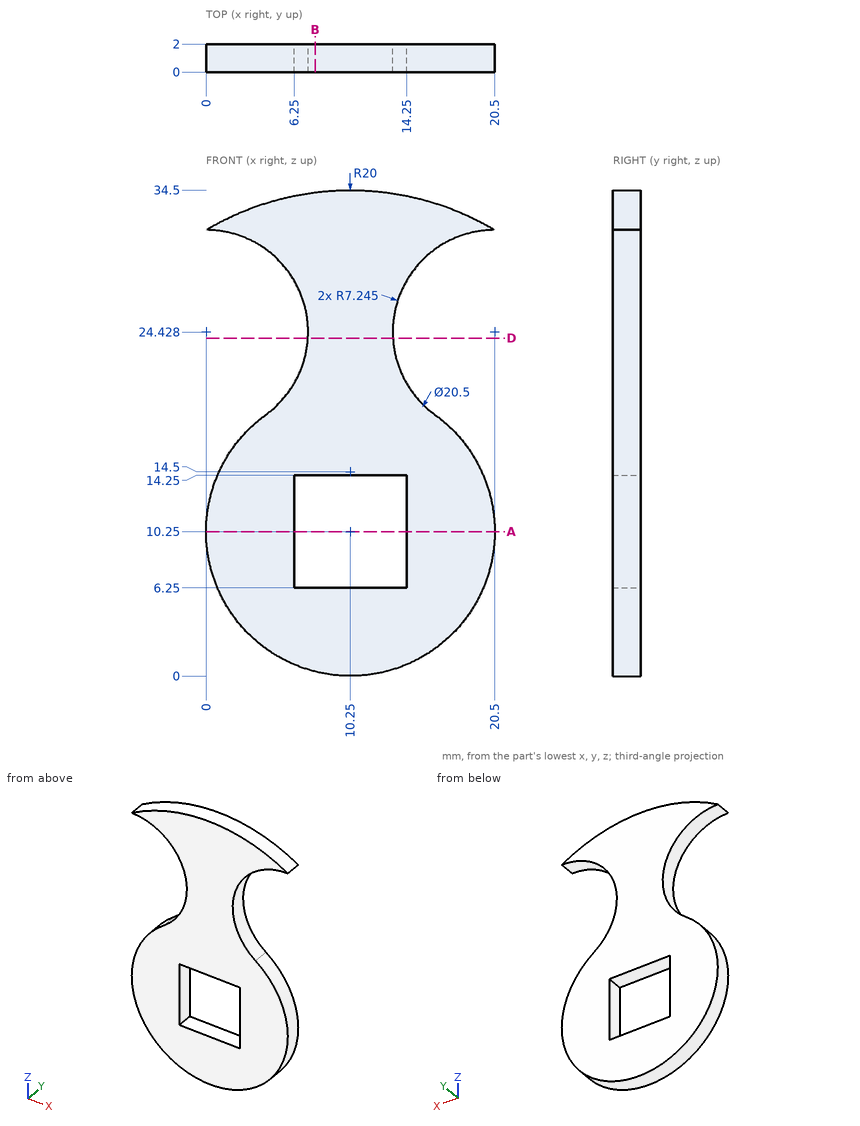
Source: three-view drawing plus pictorial views. Frame: mm from the lowest corner of the part. Round coordinates to 2 decimals unless told otherwise and drop trailing zeros. Order: outer loops, then holes, each group sorted by start corner. A loop starts at its lowest first (then second) coordinate and runs counter-clockwise, first axis right, second up. Notation, with made-up numbers: (35, 61) -> (61, 61) arc R19 ccw to (61, 80) -> close; hole circle Ø9 at (47.25, 35.25). An arc over 180 degrees is marked (long way). Use one line per item in the form item = value. Start each with the question number.
1. Cut plane A-A (z = 10.25). Return the cut outline in (x, y), then the cut area to 3 significant figures.
2. Cut plane D-D (z = 24). Return the cut outline in (x, y).
3. Cut plane B-B (x = 7.75). Return the cut outline in (y, z).
4. Pin query (flat end, axial travel): pin 1 Ø1 at (y, z) = (0.5, 28) entering from +X; pin 2 Ø1 at (y, z) = (1.5, 8.5) entering from +X; pin 3 Ø1 at (y, z) = (0.5, 27) entering from -X; pin 4 Ø0.6 at (y, z) = (1, 10.5) entering from -X. Return the tip coordinate at first contact, or that it passes through.
5. Line query: probe 1 along Z at (x, y) = (12, 0.8); probe 2 along Z at (x, y) = (9.5, 1.4); probe 3 along X at (y, z) = (0.6, 28) (1 decimal). Output: solid intervals per line, ascending.
Solution:
q1.outline = (0, 0) -> (6.25, 0) -> (6.25, 2) -> (0, 2) -> close; (14.25, 0) -> (20.5, 0) -> (20.5, 2) -> (14.25, 2) -> close
q1.area = 25.0 mm^2
q2.outline = (7.23, 0) -> (13.27, 0) -> (13.27, 2) -> (7.23, 2) -> close
q3.outline = (0, 0.31) -> (2, 0.31) -> (2, 6.25) -> (0, 6.25) -> close; (0, 14.25) -> (2, 14.25) -> (2, 34.34) -> (0, 34.34) -> close
q4.pin_1 = 14.51
q4.pin_2 = 20.42
q4.pin_3 = 6.56
q4.pin_4 = 0
q5.probe_1 = 0.15 to 6.25, 14.25 to 34.42
q5.probe_2 = 0.03 to 6.25, 14.25 to 34.49
q5.probe_3 = 6.3 to 14.2
